Input: part model. Units: mm. Frame: model coordinates. A direction names the side the tool comes from. Give positions to 0.01 mm unless a question says otherwise; leave off trailing zeros. Loops run counter-clockwise (first coordinate to the right, second up) from the corner with the lowest first, then second, coordinate; pieces in that order, holes last. Notation, with made-up numbers: (-32, 82) - (-24, 82) arc R19 cw to (-24, 93) - close; hole circle Ø4 at (79.5, -20). An arc over 180 degrees is marked (long way). One line per item, written item: value.
from build123d import *

# Parameters (mm, degrees)
SKETCH_W     = 33
SKETCH_H     = 17
SKETCH_R     = 2.25
PAD_DEPTH    = 6.5
SKETCH001_R  = 4.5
POCKET_DEPTH = 2.5
FILLET_R     = 1.5


with BuildPart() as part:
    # Sketch → Pad (new body)
    with BuildSketch(Plane.XY):
        with Locations((16.5, 8.5)):
            Rectangle(SKETCH_W, SKETCH_H)
        with Locations((6.5, 8.5)):
            Circle(SKETCH_R, mode=Mode.SUBTRACT)
        with Locations((26.5, 8.5)):
            Circle(SKETCH_R, mode=Mode.SUBTRACT)
    extrude(amount=PAD_DEPTH)

    # Sketch001 (on Face8 of Pad) → Pocket (cut)
    with BuildSketch(Plane.XY.offset(6.5)):
        with Locations((6.5, 8.5)):
            Circle(SKETCH001_R)
        with Locations((26.5, 8.5)):
            Circle(SKETCH001_R)
    extrude(amount=-POCKET_DEPTH, mode=Mode.SUBTRACT)

    # Fillet
    fillet_edges = [part.edges().sort_by_distance(p)[0] for p in [
        (33, 8.5, 6.5),
        (0, 8.5, 6.5),
    ]]
    fillet(fillet_edges, radius=FILLET_R)


solid = part.part
Item 1: Access query for faces 1 (the face through (4, 8, 4)), 2 (the face through (33, 8, 2)). Directions: +Z, -Z, +X, -X, +Y, -Y. A direction counts if a zero-diameter tool reaches every point of the face in a straight line with its end or side. Return the directions, or none.
Verdict:
face 1: +Z
face 2: +Z, -Z, +X, +Y, -Y
Item 2: Section B-B, the plane y = 8.5. Output: boundary loops of the cut face in (x, z), and give its area (3 significant figures).
Verdict:
outline: (0, 0) - (4.25, 0) - (4.25, 4) - (2, 4) - (2, 6.5) - (1.5, 6.5) arc R1.5 ccw to (0, 5) - close; (8.75, 0) - (24.25, 0) - (24.25, 4) - (22, 4) - (22, 6.5) - (11, 6.5) - (11, 4) - (8.75, 4) - close; (28.75, 0) - (33, 0) - (33, 5) arc R1.5 ccw to (31.5, 6.5) - (31, 6.5) - (31, 4) - (28.75, 4) - close
area: 133 mm^2
Item 3: Draft query along Y for faces 3 (the face through (16, 17, 3)), 4 (the face through (27.71, 10.397, 1.972)), 5 (the face through (32.55, 8.62, 6.07)), 6 (the face through (16, 0, 3)). Return one class per face: pulls with the +Y half, pulls with the -Y half, needs draft (parallel to the pull), parting line crosses it, or undercut.
Verdict:
face 3: pulls with the +Y half
face 4: undercut
face 5: needs draft
face 6: pulls with the -Y half
Item 4: Section A-A, the plane x = 6.5. Output: boundary loops of the cut face in (y, z).
Verdict:
outline: (0, 0) - (6.25, 0) - (6.25, 4) - (4, 4) - (4, 6.5) - (0, 6.5) - close; (10.75, 0) - (17, 0) - (17, 6.5) - (13, 6.5) - (13, 4) - (10.75, 4) - close
Item 5: Section D-D, the plane y = 11.25. Output: boundary loops of the cut face in (x, z).
Verdict:
outline: (0, 0) - (33, 0) - (33, 5) arc R1.5 ccw to (31.5, 6.5) - (30.06, 6.5) - (30.06, 4) - (22.94, 4) - (22.94, 6.5) - (10.06, 6.5) - (10.06, 4) - (2.94, 4) - (2.94, 6.5) - (1.5, 6.5) arc R1.5 ccw to (0, 5) - close
Item 6: Material intervals for L1, parallel to X at y = 8.5, z = 3.1; L2, parallel to Y at x = 26.5, z = 2.6; L3, parallel to Y at x = 6.5, z = 5.6, sorted ascending.
Verdict:
L1: x = 0 to 4.25, 8.75 to 24.25, 28.75 to 33
L2: y = 0 to 6.25, 10.75 to 17
L3: y = 0 to 4, 13 to 17
Item 7: Pin query (flat end, axial travel): P1, Ø2.5, axis at x = 26, y = 7, coming from the +Z side. Return the tip coordinate at first contact, or that it passes through.
Verdict:
P1: stops at z = 4
Item 8: Section C-C, the plane z = 0.5. Output: boundary loops of the cut face in (x, y).
Verdict:
outline: (0, 0) - (33, 0) - (33, 17) - (0, 17) - close; hole circle Ø4.5 at (6.5, 8.5); hole circle Ø4.5 at (26.5, 8.5)
